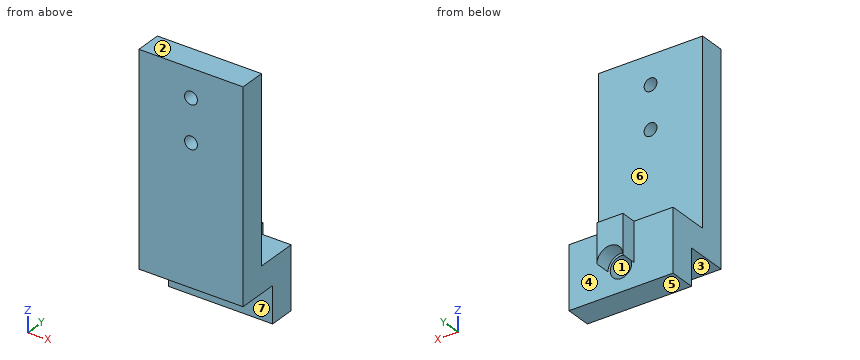
Autodesk Inventor part; units mm, degrees
ref_plane "YZ Plane" through (0, 0, 0) normal (1, 0, 0) x (0, 1, 0)
ref_plane "XZ Plane" through (0, 0, 0) normal (0, 1, 0) x (-1, 0, 0)
ref_plane "XY Plane" through (0, 0, 0) normal (0, 0, 1) x (1, 0, 0)
sketch "Skizze1" plane through (0, 0, 0) normal (1, 0, 0) x (0, 1, 0)
  line L0 (8, 0) -> (0, 0)
  line L1 (0, 0) -> (0, 35)
  line L2 (0, 35) -> (-5, 35)
  line L3 (-5, 35) -> (-5, -5)
  line L4 (-5, -5) -> (3, -5)
  line L5 (3, -5) -> (3, -12)
  line L6 (3, -12) -> (8, -12)
  line L7 (8, -12) -> (8, 0)
  dimension "d0" = 5
  dimension "d1" = 35
  dimension "d2" = 5
  dimension "d3" = 5
  dimension "d4" = 12
  dimension "d5" = 8
extrude "Extrusion1" add sketch "Skizze1" along normal mid plane 20
sketch "Skizze2" plane through (-10, 8, 0) normal (0, 1, 0) x (1, 0, 0)
  line L0 (20, 0) -> (0, 0)
  line L1 (12.5, 0) -> (7.5, 0)
  line L2 (7.5, 0) -> (7.5, 7.5)
  line L3 (7.5, 7.5) -> (12.5, 7.5)
  line L4 (12.5, 7.5) -> (12.5, 0)
  circle A0 centre (10, 7.5) radius 2.5
  point P0 (10, 0)
  point P1 (10, 0)
  dimension "d8" = 5
  dimension "d9" = 7.5
  dimension "d10" = 5
extrude "Extrusion2" add sketch "Skizze2" along normal blind 3 contours L0 L2 A0 L4
sketch "Skizze3" plane through (-10, 8, -12) normal (0, 1, 0) x (1, 0, 0)
  arc A0 (7.5, -4.5) -> (12.5, -4.5) centre (10, -4.5) ccw
  point P0 (10, -12)
hole "Bohrung1" at (0, 8, -7.5) direction (0, -1, 0) diameter 4.134 end through all
sketch "Skizze4" plane through (-10, 0, 35) normal (0, 1, 0) x (1, 0, 0)
  line L0 (10, 35) -> (10, 0) construction
  line L1 (0, 0) -> (20, 0)
  line L2 (20, 35) -> (0, 35)
  point P0 (10, 5.45)
  point P1 (10, 13.6)
  dimension "d20" = 21.4
  dimension "d21" = 29.55
hole "Bohrung2" at (0, 0, 29.55) at (0, 0, 21.4) direction (0, -1, 0) diameter 2.459 end through all
properties part number "Nozzle_Brush_Holder_slim"
Can you work these out from the model? Positions are in its coordinate system, mm. Face numbers are marked on the shaded views. A direction names the side the tool comes from. Give positions to 0.01 mm unless a question says otherwise; leave off trailing zeros. Loops run counter-clockwise (first coordinate to the right, second up) from the corner with the lowest first, then second, coordinate; pieces in that order, holes last. Notation, with made-up numbers: (48.25, 64.5) - (70.25, 64.5) arc R30 ccw to (70.25, 90.5) - close; hole circle Ø2 at (-14, 38.25). An arc over 180 degrees is marked (long way). Return JSON: item names as keys, results as strings.
1. I want a section at C-C on y = -2. Please give me the cut outline in (x, z), and give its area (4 significant figures).
Output values:
{"outline": "(-10, -5) - (10, -5) - (10, 35) - (-10, 35) - close; hole circle Ø2.46 at (0, 21.4); hole circle Ø2.46 at (0, 29.55)", "area": "790.5 mm²"}
2. I want a section at A-A on z = 21.4. Please give me the cut outline in (x, y), and give its area (3 significant figures).
Output values:
{"outline": "(-10, -5) - (-1.23, -5) - (-1.23, 0) - (-10, 0) - close; (1.23, -5) - (10, -5) - (10, 0) - (1.23, 0) - close", "area": "87.7 mm²"}
3. I want a section at D-D on x = 0. Please give me the cut outline in (y, z), and give its area (3 significant figures).
Output values:
{"outline": "(-5, -5) - (3, -5) - (3, -5.43) - (8, -5.43) - (8, -5) - (11, -5) - (11, 0) - (0, 0) - (0, 20.17) - (-5, 20.17) - close; (-5, 22.63) - (0, 22.63) - (0, 28.32) - (-5, 28.32) - close; (-5, 30.78) - (0, 30.78) - (0, 35) - (-5, 35) - close; (3, -12) - (8, -12) - (8, -9.57) - (3, -9.57) - close", "area": "245 mm²"}
4. For the marked faces 5, 6 and 7, which set-ups out of +Z, -Z, +X, -X, +Y, -Y let a thin tool reach every point of the face, with its end or its side?
Output values:
{"face 5": "-Z, +X, -X, +Y, -Y", "face 6": "+Z, +X, -X, +Y", "face 7": "-Z, +X, -X, -Y"}
5. If I drill on line 1 (Z direction, x = 0, y = -3.1); line 2 (X direction, y = -2.65, z = 29.55); line 3 (Z direction, x = 0, y = 6.8), over which ranges is the centre line in solid material (lowest first)?
Output values:
{"line 1": "z = -5 to 20.17, 22.63 to 28.32, 30.78 to 35", "line 2": "x = -10 to -1.23, 1.23 to 10", "line 3": "z = -12 to -9.57, -5.43 to 0"}
6. I'm going to push flat-ended pins straight in: pin 1 Ø4 at (x, y) = (3, -3) entering from -Z; pin 2 Ø2 at (x, z) = (0, 29.55) entering from -Y; pin 3 Ø3.5 at (y, z) = (9.5, -3.5) entering from -X; pin 4 Ø3 at (x, z) = (-7, 20.5) entering from +Y. Where does each tip first touch, or does it pass through?
Output values:
{"pin 1": "stops at z = -5", "pin 2": "passes through", "pin 3": "stops at x = -10", "pin 4": "stops at y = 0"}
7. We'd pull the mould along Z, two halves only. Please class the marked faces 1, 2, 3 and 4: +Z half, -Z half, draft (parallel to the pull), parting line (faces both ways), or undercut.
Output values:
{"face 1": "undercut", "face 2": "+Z half", "face 3": "-Z half", "face 4": "draft"}
8. I want a section at B-B on x = 5.5. Please give me the cut outline in (y, z), and give its area (3 significant figures).
Output values:
{"outline": "(-5, -5) - (3, -5) - (3, -12) - (8, -12) - (8, 0) - (0, 0) - (0, 35) - (-5, 35) - close", "area": "275 mm²"}
